```python
from build123d import *

# Parameters (mm, degrees)
SKETCH2_R               = 29
BASENUT_DEPTH           = 11.2
CHAMFER1_SIZE           = 1
SKETCH3_R               = 18.688
HOLE_DEPTH              = 12.2
ENDCHAMFER_SIZE2        = 0.5
ENDCHAMFER_SIZE         = 0.866025404
ENDCHAMFER_EDGE_2_SIZE2 = 0.5
ENDCHAMFER_EDGE_2_SIZE  = 0.866025404
SLOTCUT_DEPTH           = 12.2
SLOTPAT_COUNT           = 4
LPATTERN10_COUNT        = 10
LPATTERN10_PITCH        = 0.9744


with BuildPart() as part:
    # Sketch2 → BaseNut (new body)
    with BuildSketch(Plane.XY):
        Circle(SKETCH2_R)
    extrude(amount=-BASENUT_DEPTH)

    # Chamfer1
    chamfer1_edges = [part.edges().sort_by_distance(p)[0] for p in [
        (-29, 0, 0),
        (-29, 0, -11.2),
    ]]
    chamfer(chamfer1_edges, length=CHAMFER1_SIZE)

    # Sketch3 → Hole (cut, through all)
    with BuildSketch(Plane(origin=(-17.561722019, 31.682666601, 0), x_dir=(1, 0, 0), z_dir=(0, 0, 1))):
        with Locations((17.561722019, -31.682666601)):
            Circle(SKETCH3_R)
    extrude(amount=-HOLE_DEPTH, mode=Mode.SUBTRACT)

    # EndChamfer
    endchamfer_edges = [part.edges().sort_by_distance(p)[0] for p in [
        (-18.688, 0, -11.2),
    ]]
    chamfer(endchamfer_edges, length=ENDCHAMFER_SIZE, length2=ENDCHAMFER_SIZE2)

    # EndChamfer edge 2
    endchamfer_edge_2_edges = [part.edges().sort_by_distance(p)[0] for p in [
        (-18.688, 0, 0),
    ]]
    chamfer(endchamfer_edge_2_edges, length=ENDCHAMFER_EDGE_2_SIZE, length2=ENDCHAMFER_EDGE_2_SIZE2)

    # Sketch4 → SlotCut (cut, through all)
    with BuildSketch(Plane(origin=(-28.84840977, 49.266341409, 0), x_dir=(1, 0, 0), z_dir=(0, 0, 1))):
        with BuildLine():
            Line((25.84840977, -20.421931205), (25.84840977, -22.921931205))
            Line((25.84840977, -22.921931205), (31.84840977, -22.921931205))
            Line((31.84840977, -22.921931205), (31.84840977, -20.421931205))
            ThreePointArc((31.84840977, -20.421931205), (28.84840977, -20.266341409), (25.84840977, -20.421931205))
        make_face()
    slotcut = extrude(amount=-SLOTCUT_DEPTH, mode=Mode.SUBTRACT)

    # SlotPat: SlotCut ×4 about axis
    slotpat_axis = Axis((0, 0, 0), (0, 0, 1))
    for i in range(1, SLOTPAT_COUNT):
        add(slotcut.rotate(slotpat_axis, i * 360 / SLOTPAT_COUNT), mode=Mode.SUBTRACT)

    # Sketch5 → Cut-Revolve10 (revolve, cut)
    with BuildSketch(Plane(origin=(0, 0, 0), x_dir=(1, 0, 0), z_dir=(0, 1, 0))):
        Polygon((17.876, 1.272025404), (17.876, 0.460025404), (18.688, 0.460025404), (19.391212628, 0.866025404), (18.688, 1.272025404), align=None)
    cut_revolve10 = revolve(axis=Axis((0, 0, -37.301805437), (0, 0, 1)), mode=Mode.SUBTRACT)

    # LPattern10: Cut-Revolve10 ×10
    with Locations(*[(0, 0, -i * LPATTERN10_PITCH) for i in range(1, LPATTERN10_COUNT)]):
        add(cut_revolve10, mode=Mode.SUBTRACT)


solid = part.part
```
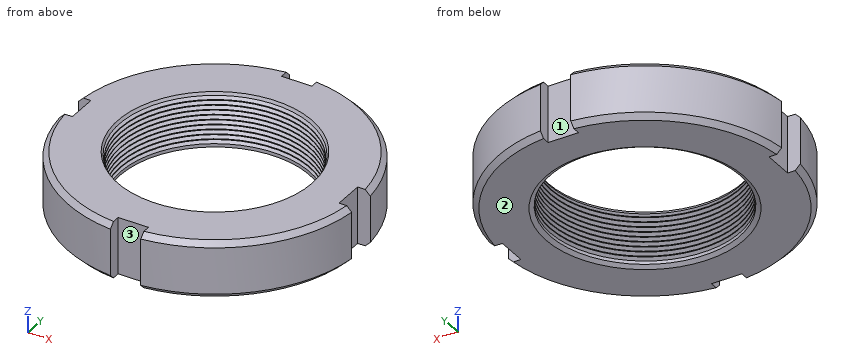
Geometry check sheet. Reference: the model listing, model coordinates, mm. Face numbers are marked on the shaded views. A direction names the side the tool comes from. Coordinates: 2 decimals unless noted, no trailing zeros.
Item 1: Go/stop test with flat-tipped pins: pin 1 Ø3 at (x, z) = (-0.5, -5) entering from +Y; pin 2 Ø6.5 at (y, z) = (-0.5, -4.5) entering from -X; pin 3 Ø22.5 at (x, y) = (0, 0) entering from +Z; pin 4 Ø5 at (y, z) = (-10, -3.5) entering from -X. Record where each tip stops, or that it passes through.
Item 2: Thickness scan on line 1 (Y direction, x = 0, z = -1.4); line 2 (X direction, y = 14, z = -5.25); line 3 (X direction, y = -4.5, z = -6.75). Record the ranges inside material, lowest first.
Item 3: Access from +Z, -Z, +X, -X, +Y, -Y to the whole of each face (thin tool, end or side, straight path). Record for the marked faces 1, 2 and 3.
Check result:
1. pin 1: stops at y = 26.34
1. pin 2: stops at x = -28.84
1. pin 3: passes through
1. pin 4: stops at x = -28.01
2. line 1: y = -26.34 to -18.69, 18.69 to 26.34
2. line 2: x = -25.4 to -12.38, 12.38 to 25.4
2. line 3: x = -28.65 to -18.79, 18.79 to 28.65
3. face 1: +Z, -Z, +Y
3. face 2: -Z, +X, -X, +Y, -Y
3. face 3: +Z, -Z, -Y
